Geometry: final body of the model. Coordinates: model frame, mm. Face numbers are marked on the shaded views. A direction names the side the tool comes from. Round coordinates to 2 decimals unless told otherwise and drop trailing zeros. Order: outer loops, then holes, each group sorted by start corner. A loop starts at its lowest first (then second) coordinate and runs counter-clockwise, first axis right, second up. Notation, with made-up numbers: (-8.75, 86) - (40.25, 86) arc R35 ccw to (40.25, 121) - close; hole circle Ø1 at (-11.5, -24). An arc over 180 degrees is marked (long way). Put each result on its own line as item: value. Start each with the question number.
(1) Section D-D (x = -2). Output: boundary loops of the cut face in (y, z), and give its area (3 significant figures).
(2) Section C-C (z = 0.35). Output: boundary loops of the cut face in (x, y).
(3) Section A-A (y = 0). Output: boundary loops of the cut face in (x, z), and give its area (3 significant figures).
(4) Material intervals for L1, parallel to Y at x = 0, z = 1.65; L2, parallel to Y at x = 0, z = 2.65; L3, parallel to X at y = -0.75, z = 2.95, sorted ascending. Write a range as [from, to].
(5) Pin query (flat end, axial travel): P1, Ø1.5, axis at x = 2, y = 3, coming from the -Z side; P2, Ø1, axis at y = -1.5, z = 3, coming from the -X side; P3, Ø1, axis at y = 2, z = 1.5, coming from the +X side; P4, Ø1.9, axis at x = 0, y = 0, coming from the -Z side. Return the tip coordinate at first contact, or that it passes through.
(6) Pull-direction query (Y, two-part tool) for the marked faces 3, 4 and 5; classes: released by +Y, released by -Y, zero draft, split by the parting line, or undercut.
(7) Access query for the marked faces 1 and 2. Directions: +Z, -Z, +X, -X, +Y, -Y. A direction counts if a zero-diameter tool reaches every point of the face in a straight line with its end or side. Return the directions, or none.
Autodesk Inventor part; units mm, degrees
ref_plane "YZ Plane" through (0, 0, 0) normal (1, 0, 0) x (0, 1, 0)
ref_plane "XZ Plane" through (0, 0, 0) normal (0, 1, 0) x (-1, 0, 0)
ref_plane "XY Plane" through (0, 0, 0) normal (0, 0, 1) x (1, 0, 0)
sketch "Skizze1" plane through (0, 0, 0) normal (0, 0, 1) x (1, 0, 0)
  circle A0 centre (0, 0) radius 3
  dimension "d0" = 6
extrude "Extrusion1" add sketch "Skizze1" along normal blind 2.5
sketch "Skizze2" plane through (0, 0, 2.5) normal (0, 0, 1) x (1, 0, 0)
  circle A0 centre (0, 0) radius 4
  dimension "d3" = 8
extrude "Extrusion2" add sketch "Skizze2" along normal blind 1
hole "Bohrung1" at (0, 0, 0) direction (0, 0, 1) diameter 3.242 end through all
properties part number "MutterMitUScheibe"
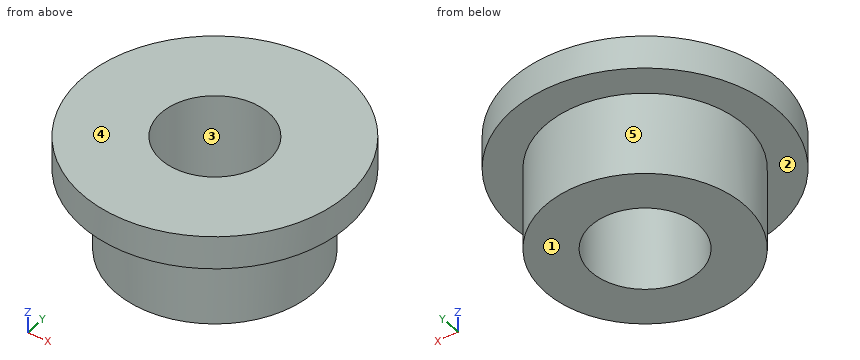
Checks:
1. outline: (-3.46, 2.5) - (-2.24, 2.5) - (-2.24, 0) - (2.24, 0) - (2.24, 2.5) - (3.46, 2.5) - (3.46, 3.5) - (-3.46, 3.5) - close
1. area: 18.1 mm²
2. outline: circle Ø6 at (0, 0); hole circle Ø3.24 at (0, 0)
3. outline: (-4, 2.5) - (-3, 2.5) - (-3, 0) - (-1.62, 0) - (-1.62, 3.5) - (-4, 3.5) - close; (1.62, 0) - (3, 0) - (3, 2.5) - (4, 2.5) - (4, 3.5) - (1.62, 3.5) - close
3. area: 11.7 mm²
4. L1: y = [-3, -1.62], [1.62, 3]
4. L2: y = [-4, -1.62], [1.62, 4]
4. L3: x = [-3.93, -1.44], [1.44, 3.93]
5. P1: stops at z = 0
5. P2: stops at x = -3.87
5. P3: stops at x = 2.6
5. P4: passes through
6. face 3: undercut
6. face 4: zero draft
6. face 5: split by the parting line
7. face 1: -Z, +X, -X, +Y, -Y
7. face 2: -Z
